Can you work these out from the model? Positions are in its coordinate system, mm. Face numbers are marked on the shaded views. A direction names the side the tool comes from. Coordinates: 2 decimals unless noted, no trailing zeros. Loops run counter-clockwise (first coordinate to the right, second up) from the corner with the lowest first, then second, coordinate; pieces in that order, holes last.
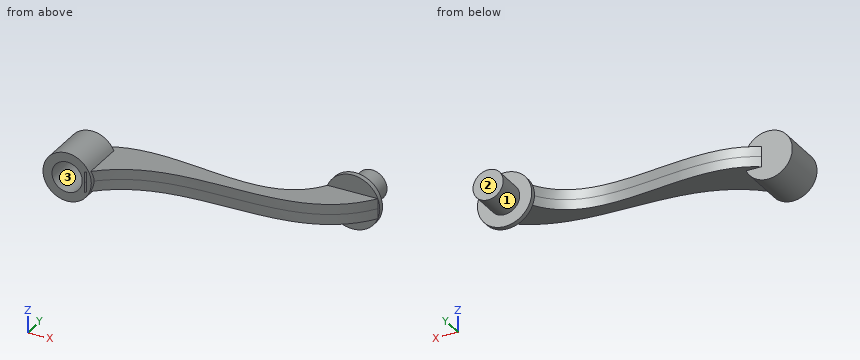
```python
from build123d import *

# Parameters (mm, degrees)
BOSS_EXTRUDE1_START = 7.5
SKETCH1_R           = 12
SKETCH1_R_2         = 7.5005
BOSS_EXTRUDE1_DEPTH = 20
BOSS_EXTRUDE2_DEPTH = 5
BOSS_EXTRUDE3_START = 27.5
SKETCH1_2_R         = 12
SKETCH1_2_R_2       = 7.5005
BOSS_EXTRUDE3_DEPTH = 2.5
SKETCH3_R           = 13.462912018
BOSS_EXTRUDE4_DEPTH = 2.5
SKETCH5_R           = 7.5
BOSS_EXTRUDE5_DEPTH = 15


with BuildPart() as part:
    # Sketch1 → Boss-Extrude1 (new body)
    with BuildSketch(Plane(origin=(0, 0, 0), x_dir=(1, 0, 0), z_dir=(0, 1, 0)).offset(BOSS_EXTRUDE1_START)):
        Circle(SKETCH1_R)
        Circle(SKETCH1_R_2, mode=Mode.SUBTRACT)
    extrude(amount=BOSS_EXTRUDE1_DEPTH)

    # Sketch2 → Boss-Extrude2 (add, symmetric)
    with BuildSketch(Plane.XY):
        with BuildLine():
            Line((0, 27.5), (8.9613053, 27.5))
            Line((8.9613053, 27.5), (8.9613053, 6.915260629))
            add(Edge.make_bspline(
                [(8.9613053, 6.915260629), (42.430030167, 43.623802214), (104.826512854, 5.893256195), (132.347009744, 47.5)],
                knots=[0, 0, 0, 0, 1, 1, 1, 1], degree=3))
            Line((132.347009744, 47.5), (107.347009744, 47.5))
            add(Edge.make_bspline(
                [(0, 27.5), (29.095772849, 52.440117374), (86.574153169, 13.532011579), (107.347009744, 47.5)],
                knots=[0, 0, 0, 0, 1, 1, 1, 1], degree=3))
        make_face()
    extrude(amount=BOSS_EXTRUDE2_DEPTH, both=True)

    # Sketch1<2> → Boss-Extrude3 (add)
    with BuildSketch(Plane(origin=(0, 0, 0), x_dir=(1, 0, 0), z_dir=(0, 1, 0)).offset(BOSS_EXTRUDE3_START)):
        Circle(SKETCH1_2_R)
        Circle(SKETCH1_2_R_2, mode=Mode.SUBTRACT)
        Circle(SKETCH1_2_R_2)
    extrude(amount=BOSS_EXTRUDE3_DEPTH)

    # Sketch3 → Boss-Extrude4 (add)
    with BuildSketch(Plane(origin=(0, 47.5, 0), x_dir=(1, 0, 0), z_dir=(0, 1, 0))):
        with Locations((119.847009744, 0)):
            Circle(SKETCH3_R)
    extrude(amount=BOSS_EXTRUDE4_DEPTH)

    # Sketch5 → Boss-Extrude5 (add)
    with BuildSketch(Plane(origin=(0, 50, 0), x_dir=(1, 0, 0), z_dir=(0, 1, 0))):
        with Locations((119.847009744, 0)):
            Circle(SKETCH5_R)
    extrude(amount=BOSS_EXTRUDE5_DEPTH)


solid = part.part
```
Item 1: Suppose I cut it at A-A, the plane x = 0. Please give me the cut outline in (y, z), plus the area to 3 significant figures.
Results are:
outline: (7.5, -12) - (30, -12) - (30, 12) - (7.5, 12) - (7.5, 7.5) - (27.5, 7.5) - (27.5, -7.5) - (7.5, -7.5) - close
area: 240 mm2
Item 2: On a 3-axis mill with a long thin cutter (end or side, diameter ignored), from which of +Z, -Z, +X, -X, +Y, -Y can I reach the whole of each face in a straight line? I mean the marked faces 1, 2 and 3. Say none if no direction works.
Results are:
face 1: +Y
face 2: +Z, -Z, +X, -X, +Y
face 3: -Y
Item 3: I need wall thicknesses on line 1 along Z through (x, y) = (0, 14.25); line 2 along Y through (x, z) = (-1, 7.25); line 3 along Y through (x, z) = (7, 9). Which ranges of each line are inside material? Lowest first, please.
Results are:
line 1: z = -12 to -7.5, 7.5 to 12
line 2: y = 27.5 to 30
line 3: y = 7.5 to 30
Item 4: Suppose I cut it at B-B, the plane y = 60.5. Please give me the cut outline in (x, z), plus the area to 3 significant figures.
Results are:
outline: circle Ø15 at (119.85, 0)
area: 177 mm2
Item 5: I'm going to push flat-ended pins straight in: P1, Ø7, axis at x = -5.5, z = 2.5, coming from the +Y side; P2, Ø1.5, axis at y = 36, z = -7.5, coming from the +X side; P3, Ø10, axis at x = 63.5, z = -9.5, coming from the +Y side; P4, Ø13.5, axis at x = 0, z = 0, coming from the -Y side. Where does each tip first touch, or does it pass through?
Results are:
P1: stops at y = 30
P2: passes through
P3: stops at y = 33.62
P4: stops at y = 27.5
